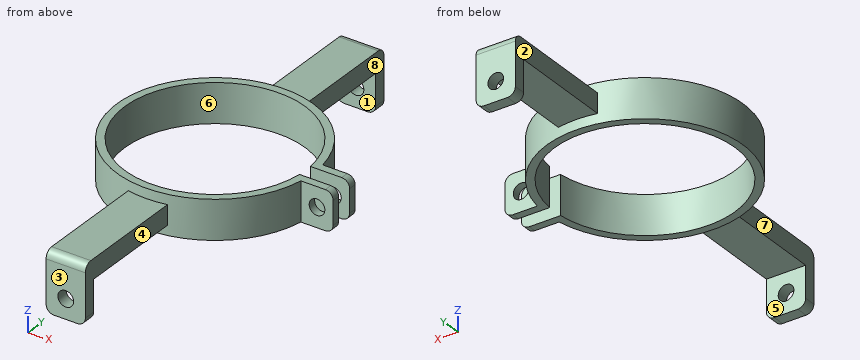
Autodesk Inventor part; units mm, degrees
ref_plane "Work Plane1" through (24.6779, 24, 0) normal (0, 1, 0) x (1, 0, 0)
ref_plane "Work Plane2" through (0, 0, 0) normal (0.7071, -0.7071, 0) x (0, 0, -1)
ref_plane "XY Plane" through (0, 0, 0) normal (0, 0, 1) x (1, 0, 0)
sketch "Sketch1" plane through (0, 0, 0) normal (0, 0, 1) x (1, 0, 0)
  arc A0 (22.9129, 2) -> (22.9129, -2) centre (0, 0) ccw
  arc A1 (24.6779, 4) -> (24.6779, -4) centre (0, 0) ccw
  line L0 (22.9129, 2) -> (24.9199, 2)
  line L1 (22.9129, -2) -> (24.9199, -2)
  line L2 (24.9199, 2) -> (32.9199, 2)
  line L3 (32.9199, 2) -> (32.9199, 4)
  line L4 (32.9199, 4) -> (24.6779, 4)
  line L5 (24.9199, -2) -> (32.9199, -2)
  line L6 (32.9199, -2) -> (32.9199, -4)
  line L7 (32.9199, -4) -> (24.6779, -4)
  dimension "d0" = 46
  dimension "d1" = 50
  dimension "d7" = 2
  dimension "d9" = 2
extrude "Extrusion1" add sketch "Sketch1" against normal blind 10
sketch "Sketch2" plane through (24.6779, 4, 0) normal (0, 1, 0) x (1, 0, 0)
  line L0 (8.2419, 0) -> (0, 0)
  line L1 (8.2419, 0) -> (8.2419, 10)
  line L2 (0, 10) -> (8.2419, 10)
  line L3 (0, 0) -> (0, 10)
  circle A0 centre (4.121, 5) radius 2
  point P0 (-24.6779, 0)
  dimension "d12" = 4
extrude "Extrusion2" cut sketch "Sketch2" against normal blind 8.5 contours A0
ref_plane "Work Plane1" through (24.6779, 24, 0) normal (0, 1, 0) x (1, 0, 0)
sketch "Sketch3" plane through (24.6779, 24, 0) normal (0, 1, 0) x (1, 0, 0)
  line L0 (-24.6779, 0) -> (-24.6779, 10)
  line L1 (-19.6779, 7.5) -> (-29.6779, 7.5)
  line L2 (-29.6779, 2.5) -> (-19.6779, 2.5)
  line L3 (-19.6779, 2.5) -> (-19.6779, 7.5)
  line L4 (-29.6779, 2.5) -> (-29.6779, 7.5)
  point P0 (-24.6779, 5)
extrude "Extrusion3" add sketch "Sketch3" along normal blind 27.5
sketch "Sketch4" plane through (5, 24.4949, -6) normal (1, 0, 0) x (0, 0, -1)
  line L0 (1.5, 27.0051) -> (-3.5, 27.0051)
  line L1 (-3.5, 27.0051) -> (11.5, 27.0051)
  line L2 (11.5, 27.0051) -> (11.5, 30.0051)
  line L3 (11.5, 30.0051) -> (-3.5, 30.0051)
  line L4 (-3.5, 30.0051) -> (-3.5, 27.0051)
  point P0 (-6, -24.4949)
  dimension "d27" = 15
  dimension "d28" = 3
extrude "Extrusion4" add sketch "Sketch4" against normal blind 10
ref_plane "Work Plane2" through (0, 0, 0) normal (0.7071, -0.7071, 0) x (0, 0, -1)
sketch "Sketch5" plane through (5, 54.5, -2.5) normal (0, 1, 0) x (1, 0, 0)
  circle A0 centre (-5, 10) radius 2
  dimension "d29" = 4
extrude "Extrusion5" cut sketch "Sketch5" against normal blind 4
mirror "Mirror2" about plane through (0, 0, 0) normal (0, 1, 0) of "Extrusion4", "Extrusion5", "Extrusion3"
fillet "Fillet1" radius 2 10 edges at (0, 54.5, -2.5) (5, 53, -17.5) (-5, 53, -17.5) (5, -53, -17.5) (-5, -53, -17.5) (0, -54.5, -2.5) (32.9199, 3, 0) (32.9199, 3, -10) (32.9199, -3, 0) (32.9199, -3, -10)
properties part number "SupportBracket_BilgePumpMotor" material "ABS Plastic"
CAD build for the part. Positions are in the model's coordinates, mm. Face numbers are marked on the shaded views. A direction names the side the tool comes from. Coordinates: 2 decimals unless noted, no trailing zeros. Write each loop counter-clockwise with the first axis right and the second up, starting at its lowest first coordinate (ties: lowest second). Pieces come first, ordered by that corner, then holes.
(1) 3-axis set-ups, long thin cutter, end or side, ignore diameter. For the marked faces 4, 5, 6, 7 and 8: which of +Z, -Z, +X, -X, +Y, -Y reach the whole face in a straight line?
(2) Cut at A-A, the plane x = 0. Count the separate pieces of the cut face and the enclosed holes in it, and give its area (3 significant figures).
(3) Flat gauge pins, fed straight in: pin 1 (5 mm diameter, centred on x = -1.5, y = 40, fed in from +Z); pin 2 (6 mm diameter, centred on y = 16.5, z = -14, fed in from -X); pin 3 (5 mm diameter, centred on x = 28.8, z = -5, fed in from -Y); pin 4 (6.5 mm diameter, centred on x = 0, z = -12.5, fed in from -Y). Where does each tip first touch, or does it go through?
(4) Drill centre lines: probe 1 along Y at (x, z) = (4, -13.5); probe 2 along Y at (x, z) = (0, -5.5); probe 3 along X at (y, z) = (-2.9, -5). Where is each one in solid material? Low to high.
(5) Cut at D-D, the plane x = 29. List the corners of the cut face in (y, z).
(6) Cut at C-C, the plane x = 16. List the corners of the cut face in (y, z).
(7) Two-plate mould, pull along Y, no slides. Class the marked faces 1, 2 and 3: +Y half, -Y half, draft (parallel to the pull), parting line (faces both ways), or undercut.
(8) Cut at B-B, the plane z = -12.5. List the corners of the cut face in (x, y), and give its area (3 significant figures).
Geometry says:
1. face 4: +Z, -Z, +X, -Y
1. face 5: -Z, +X, -X
1. face 6: +Z, -Z
1. face 7: +Z, -Z, -X, -Y
1. face 8: +Z, -Z, +X, +Y
2. separate pieces: 4
2. enclosed holes: 0
2. area: 369 mm2
3. pin 1: stops at z = -2.5
3. pin 2: passes through
3. pin 3: stops at y = -4
3. pin 4: stops at y = -54.5
4. probe 1: y = -54.5 to -51.5, 51.5 to 54.5
4. probe 2: y = -54.5 to -23, 23 to 54.5
4. probe 3: x = -24.83 to -22.82, 22.82 to 26.8, 30.8 to 32.92
5. outline: (-4, -10) - (-2, -10) - (-2, -6.99) - (-4, -6.99) - close; (-4, -3.01) - (-2, -3.01) - (-2, 0) - (-4, 0) - close; (2, -10) - (4, -10) - (4, -6.99) - (2, -6.99) - close; (2, -3.01) - (4, -3.01) - (4, 0) - (2, 0) - close
6. outline: (-19.21, -10) - (-16.52, -10) - (-16.52, 0) - (-19.21, 0) - close; (16.52, -10) - (19.21, -10) - (19.21, 0) - (16.52, 0) - close
7. face 1: undercut
7. face 2: draft
7. face 3: -Y half
8. outline: (-5, -54.5) - (-2, -54.5) - (-2, -51.5) - (-5, -51.5) - close; (-5, 51.5) - (-2, 51.5) - (-2, 54.5) - (-5, 54.5) - close; (2, -54.5) - (5, -54.5) - (5, -51.5) - (2, -51.5) - close; (2, 51.5) - (5, 51.5) - (5, 54.5) - (2, 54.5) - close
8. area: 36.0 mm2
